```python
from build123d import *

# Parameters (mm, degrees)
SKETCH1_R           = 2
SKETCH1_R_2         = 4
BOSS_EXTRUDE1_DEPTH = 11
CUT_EXTRUDE1_DEPTH  = 6
FILLET2_R           = 14
M4_TAPPED_HOLE1_D   = 3.3


with BuildPart() as part:
    # Sketch1 → Boss-Extrude1 (new body)
    with BuildSketch(Plane(origin=(0, 0, 0), x_dir=(1, 0, 0), z_dir=(0, 1, 0))):
        with BuildLine():
            Line((0, 20), (-100, 20))
            Line((-100, 20), (-100, -5))
            Line((-100, -5), (-100, -20))
            Line((-100, -20), (0, -20))
            ThreePointArc((0, -20), (14.142135607, -14.14213564), (20, -4.7e-08))
            ThreePointArc((20, -4.7e-08), (14.14213564, 14.142135607), (0, 20))
        make_face()
        with Locations(Location((-90, -10, 0), (0, 0, 270))):
            Circle(SKETCH1_R, mode=Mode.SUBTRACT)
        with Locations(Location((-65, -10, 0), (0, 0, 270))):
            Circle(SKETCH1_R, mode=Mode.SUBTRACT)
        with Locations(Location((-90, 10, 0), (0, 0, 270))):
            Circle(SKETCH1_R, mode=Mode.SUBTRACT)
        with Locations(Location((-65, 10, 0), (0, 0, 270))):
            Circle(SKETCH1_R, mode=Mode.SUBTRACT)
        with Locations(Location((0, 0, 0), (0, 0, 270))):
            Circle(SKETCH1_R_2, mode=Mode.SUBTRACT)
    extrude(amount=BOSS_EXTRUDE1_DEPTH)

    # Sketch4 → Cut-Extrude1 (cut)
    with BuildSketch(Plane(origin=(0, 11, 0), x_dir=(1, 0, 0), z_dir=(0, 1, 0))):
        with BuildLine():
            Line((-28.111385594, 20), (-100, 20))
            Line((-100, 20), (-100, -20))
            Line((-100, -20), (-28.111385594, -20))
            ThreePointArc((-28.111385594, -20), (-34.5, 0), (-28.111385594, 20))
        make_face()
    extrude(amount=-CUT_EXTRUDE1_DEPTH, mode=Mode.SUBTRACT)

    # Fillet2
    # the kernel refuses this fillet: 14 mm, written as the material it adds along each edge
    with BuildSketch(Plane(origin=(0, 5, 0), x_dir=(-0.1193853688936188, 0, 0.9928479912323611), z_dir=(0.9928479912323611, 0, 0.1193853688936188))) as fillet2_piece_1_section:
        with BuildLine():
            CenterArc((45.989125293, -14), FILLET2_R, 90, 55.150095421)
            Line((34.5, -6), (34.270217494, -5.84))
            ThreePointArc((34.270217494, -5.84), (34.22, -3), (34.22, 0))
            Line((34.22, 0), (34.5, 0.28))
            Line((34.5, 0.28), (45.989125293, 0.28))
            Line((45.989125293, 0.28), (45.989125293, 0))
        make_face()
    fillet2_piece_1 = revolve(axis=Axis((0, 5, 0), (0, -1, 0)), revolution_arc=166.286736379, mode=Mode.PRIVATE)
    fillet2_piece_1 = split(fillet2_piece_1, bisect_by=Plane(origin=(-35.442796837, 6.550585525, -20), z_dir=(0, 0, 1)), keep=Keep.TOP, mode=Mode.PRIVATE)
    fillet2_piece_1 = split(fillet2_piece_1, bisect_by=Plane(origin=(-35.442796837, 6.550585525, 20), z_dir=(0, 0, -1)), keep=Keep.TOP, mode=Mode.PRIVATE)
    add(fillet2_piece_1)

    # M4 Tapped Hole1 (through all)
    with Locations(Plane(origin=(0, 0, -20), x_dir=(-1, 0, 0), z_dir=(0, 0, -1))):
        with Locations((0, 5.5)):
            Hole(M4_TAPPED_HOLE1_D / 2)


solid = part.part
```
Source: CAD feature listing. Evaluate the final solid. Frame: model axes, mm. Round coordinates to 2 decimals unless told otherwise and drop trailing zeros. Loops run counter-clockwise (first coordinate to the right, second up) from the corner with the lowest first, then second, coordinate; pieces in that order, holes last.
1. Section query B-B on y = 9. Output: boundary loops of the cut face in (x, z), and give its area (3 significant figures).
2. Contact query for flat-ended pins moving along their axis: pin 1 (4.5 mm diameter, centred on x = -90, z = 10, fed in from -Y); pin 2 (6.5 mm diameter, centred on x = -90, z = -10, fed in from +Y). Output: stop coordinate, or through.
3. Section query C-C on z = 10. Give the number of separate pieces and of enclosed holes in the cut face, and give its area (3 significant figures).
4. Mould query, pull axis Z, two halves, no side actions, for faces 1 (the flat face through (-100, 2, 0)), 2 (the cylindrical face through (-63, 2, 10)), 3 (the flat face through (-40, 4, -20)). Classes: released by +Z, released by -Z, zero draft, split by the parting line, or undercut.
5. Ray query, L1, parallel to Z at x = -90, y = 2.6; L2, parallel to X at y = 3.75, z = -9.5; L3, parallel to X at y = 3.55, z = -10. Return the intervals inside material, ascending.
6. Section query D-D on x = 11. Output: boundary loops of the cut face in (y, z).
7. Section query A-A on x = -65. Output: boundary loops of the cut face in (y, z), and give its area (3 significant figures).
Answers below:
1. outline: (-30.16, -20) - (0, -20) arc R20 ccw to (0, 20) - (-30.16, 20) arc R36.19 ccw to start; hole circle Ø8 at (0, 0)
1. area: 1,950 mm2
2. pin 1: stops at y = 0
2. pin 2: stops at y = 5
3. separate pieces: 3
3. enclosed holes: 1
3. area: 861 mm2
4. face 1: zero draft
4. face 2: undercut
4. face 3: released by -Z
5. L1: z = -20 to -12, -8 to 8, 12 to 20
5. L2: x = -100 to -91.94, -88.06 to -66.94, -63.06 to 17.6
5. L3: x = -100 to -92, -88 to -67, -63 to 17.32
6. outline: (0, -16.7) - (11, -16.7) - (11, 16.7) - (0, 16.7) - close
7. outline: (0, -20) - (5, -20) - (5, -12) - (0, -12) - close; (0, -8) - (5, -8) - (5, 8) - (0, 8) - close; (0, 12) - (5, 12) - (5, 20) - (0, 20) - close
7. area: 160 mm2
